Geometry check sheet. Reference: the model listing, model coordinates, mm. A direction names the side the tool comes from. Give positions to 0.01 mm unless a question says otherwise; leave off trailing zeros. Write each loop counter-clockwise with the first axis right and the second up, starting at its lowest first coordinate (ties: lowest second). Pieces come first, ordered by that corner, then holes. Notation, with made-up numbers: (-31, 78.5) - (-8, 78.5) arc R20 ccw to (-8, 114.5) - close; hole circle Ø9 at (86, 53). An arc over 180 degrees is marked (long way). Use a Markdown table: item, result.
```python
from build123d import *

# Parameters (mm, degrees)
DODANIE_WYCI_GNI_CIE1_DEPTH = 20
ZAOKR_GLENIE2_R             = 5
WYTNIJ_WYCI_GNI_CIE1_DEPTH  = 43.884482968


with BuildPart() as part:
    # Szkic1 → Dodanie-wyciągnięcie1 (new body)
    with BuildSketch(Plane.XY):
        Polygon((-7.521041545, 0), (36.725544307, 0), (35.100945826, 5), (31.851748863, 15), (-2.647246102, 15), (-5.896443064, 5), align=None)
    extrude(amount=DODANIE_WYCI_GNI_CIE1_DEPTH)

    # Zaokrąglenie2
    zaokr_glenie2_edges = [part.edges().sort_by_distance(p)[0] for p in [
        (36.725544307, 0, 10),
        (-7.521041545, 0, 10),
        (-2.647246102, 15, 10),
        (31.851748863, 15, 10),
    ]]
    fillet(zaokr_glenie2_edges, radius=ZAOKR_GLENIE2_R)

    # Szkic2 → Wytnij-wyciągnięcie1 (cut, through all)
    with BuildSketch(Plane.XY.offset(20)):
        with BuildLine():
            Line((28.219036223, 14), (0.985466538, 14))
            ThreePointArc((0.985466538, 14), (-1.365674471, 13.236067977), (-2.818759527, 11.236067977))
            Line((-2.818759527, 11.236067977), (-2.820363357, 11.231120957))
            Line((-2.820363357, 11.231120957), (-4.491898112, 6.075264084))
            ThreePointArc((-4.491898112, 6.075264084), (-3.825121298, 2.581431863), (-0.639131943, 1))
            Line((-0.639131943, 1), (29.843634705, 1))
            ThreePointArc((29.843634705, 1), (33.079702682, 2.648858991), (33.64786077, 6.236067977))
            Line((33.64786077, 6.236067977), (32.023262289, 11.236067977))
            ThreePointArc((32.023262289, 11.236067977), (30.570177233, 13.236067977), (28.219036223, 14))
        make_face()
    extrude(amount=-WYTNIJ_WYCI_GNI_CIE1_DEPTH, mode=Mode.SUBTRACT)


solid = part.part
```
1) Section check A-A on x = 16.5. Record the boundary of the cut face in (y, z).
Working result:
| item | result |
|---|---|
| outline | (0, 0) - (1, 0) - (1, 20) - (0, 20) - close; (14, 0) - (15, 0) - (15, 20) - (14, 20) - close |
2) Section check B-B on y = 7.75. Record the boundary of the cut face in (x, z), then the cut area to 3 significant figures.
Working result:
| item | result |
|---|---|
| outline | (-5, 0) - (-3.95, 0) - (-3.95, 20) - (-5, 20) - close; (33.16, 0) - (34.21, 0) - (34.21, 20) - (33.16, 20) - close |
| area | 42.1 mm² |
3) Mould release check, pull along Y, two halves, no side actions. Record for faces 1 (the flat face through (15, 14, 10)), 2 (the flat face through (16, 14.2, 20)), 3 (the flat face through (15, 15, 10)), 4 (the cylindrical face through (33.05, 2.61, 10.14)): pulls with the +Y half, pulls with the -Y half, needs draft (parallel to the pull), parting line crosses it, or undercut.
Working result:
| item | result |
|---|---|
| face 1 | undercut |
| face 2 | needs draft |
| face 3 | pulls with the +Y half |
| face 4 | undercut |
4) Material ranges on L1, parallel to Y at x = 15.5, z = 2.5; L2, parallel to X at y = 2.5, z = 12.5; L3, parallel to X at y = 11, z = 16.5, recorded low to high. Write a range as from..to.
Working result:
| item | result |
|---|---|
| L1 | y = 0..1, 14..15 |
| L2 | x = -4.97..-3.76, 32.97..34.17 |
| L3 | x = -3.95..-2.9, 32.1..33.15 |
5) Depth check by flat-ended pin: P1, Ø2, axis at y = 13, z = 5, coming from the +X side. Enter the tip coordinate at first touch or a pass-through.
Working result:
| item | result |
|---|---|
| P1 | stops at x = 32.8 |
6) Set-up check for faces 5 (the flat face through (14, 0, 10)), 6 (the cylindrical face through (-3.856, 2.623, 10.14)): record each of +Z, -Z, +X, -X, +Y, -Y from which the full face is reachable in a straight line by a thin tool's end or side.
Working result:
| item | result |
|---|---|
| face 5 | +Z, -Z, +X, -X, -Y |
| face 6 | +Z, -Z |
